For this review, take the finished solid that the model builds, in its own axes (mm). Face numbers are marked on the shaded views. A direction names the side the tool comes from. Round coordinates to 2 decimals unless told otherwise and drop trailing zeros. Order: outer loops, then holes, each group sorted by start corner. A loop starts at its lowest first (then second) coordinate and runs counter-clockwise, first axis right, second up. Notation, with made-up numbers: M 82,66.5 L 140,66.5 A29 cw 140,99.5 Z; hole C 3,-23.5 d2. An arc over 180 degrees is marked long. Use a Markdown table: item, result.
from build123d import *

# Parameters (mm, degrees)
F0_R          = 25.4
F0_R_2        = 12.7
F1_DEPTH      = 76.2
F3_START      = -12.7
F3_DEPTH      = 12.7
F4_DEPTH      = 12.7
F4_DEPTH_BACK = 25.4
F5_DEPTH      = 12.7
F5_DEPTH_BACK = 25.4
F6_DEPTH      = 76.201


with BuildPart() as f1:
    # F0 (on Right) → F1 (new body)
    with BuildSketch(Plane.YZ):
        Circle(F0_R)
        Circle(F0_R_2, mode=Mode.SUBTRACT)
    extrude(amount=F1_DEPTH)



with BuildPart() as f3:
    # F2 (on Front) → F3 (new body)
    with BuildSketch(Plane.XZ.offset(F3_START)):
        Polygon((0, 50.8), (0, 38.1), (10.16, 38.1), align=None)
    extrude(amount=-F3_DEPTH)


with BuildPart() as f1_1:
    add(f1.part)

    add(f3.part)  # F4 merges F3
    # F2 (on Front) → F4 (join, two sides)
    with BuildSketch(Plane.XZ) as f4_sk:
        Polygon((0, 38.1), (0, 22.5723106414), (21.9132695347, 22.5723106414), (10.16, 38.1), align=None)
    extrude(amount=F4_DEPTH)
    extrude(f4_sk.sketch, amount=-F4_DEPTH_BACK)

    # F2 (on Front) → F5 (join, two sides)
    with BuildSketch(Plane.XZ) as f5_sk:
        Polygon((0, 22.5723106414), (0, 0), (38.1, 0), (21.9132695347, 22.5723106414), align=None)
    extrude(amount=F5_DEPTH)
    extrude(f5_sk.sketch, amount=-F5_DEPTH_BACK)

    # F0 (on Right) → F6 (cut, through all)
    with BuildSketch(Plane.YZ):
        Circle(F0_R_2)
    extrude(amount=F6_DEPTH, mode=Mode.SUBTRACT)


solid = f1_1.part
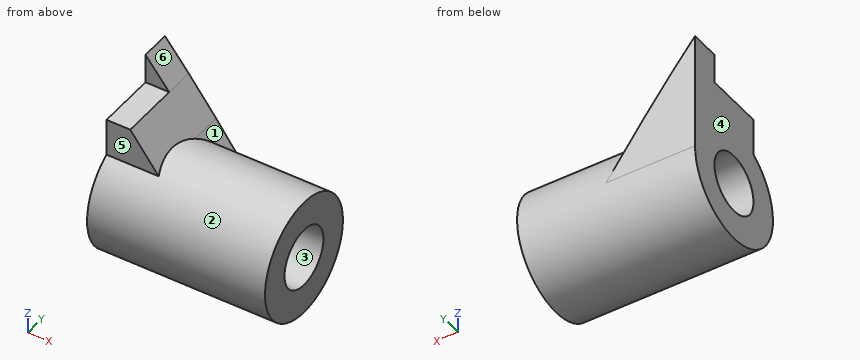
Q1. Add section A-A (y = 0). Write out the cut boundary in (x, z).
Determined:
| item | result |
|---|---|
| outline | M 0,-25.4 L 76.2,-25.4 L 76.2,-12.7 L 0,-12.7 Z; M 0,12.7 L 76.2,12.7 L 76.2,25.4 L 19.77,25.4 L 10.16,38.1 L 0,38.1 Z |
Q2. Clearance check with flat-ended pins moving along their axes: pin 1 (8 mm diameter, centred on x = 6, z = 45, fed in from -Y); pin 2 (1.5 mm diameter, centred on x = 14, z = 13.5, fed in from -Y); pin 3 (1 mm diameter, centred on x = 27.5, z = -14, fed in from -Y). State where each tip first meets the part, or that it passes through.
Determined:
| item | result |
|---|---|
| pin 1 | stops at y = 12.7 |
| pin 2 | stops at y = -21.97 |
| pin 3 | stops at y = -21.52 |
Q3. Add section D-D (z = 33). Write out the cut boundary in (x, y).
Determined:
| item | result |
|---|---|
| outline | M 0,-12.7 L 14.02,-12.7 L 14.02,25.4 L 0,25.4 Z |
Q4. Machinability: for the marked faces 5 and 6, which of the approach directions +Z, -Z, +X, -X, +Y, -Y give a long, thin tool a straight path to every point of the face, cutting with its end or side? Answer none if there is none.
Determined:
| item | result |
|---|---|
| face 5 | +Z, +X, -X, -Y |
| face 6 | +Z, +X, +Y, -Y |
Q5. Draft analysis for pull direction Z (two halves, no side actions). For the marked faces 1, 2, 3 and 4, state which applies: pulls with the +Z half, pulls with the -Z half, needs draft (parallel to the pull), parting line crosses it, or undercut.
Determined:
| item | result |
|---|---|
| face 1 | pulls with the +Z half |
| face 2 | parting line crosses it |
| face 3 | undercut |
| face 4 | needs draft |
Q6. Add section B-B (x = 62.5). Write out the cut boundary in (y, z), then the cut area to 3 significant figures.
Determined:
| item | result |
|---|---|
| outline | C 0,0 d50.8; hole C 0,0 d25.4 |
| area | 1,520 mm^2 |
Q7. Wall thickness on line 1 along Z through (x, y) = (31, 0); line 2 along Y through (x, z) = (46, -0.5); line 3 along Y through (x, z) = (9.5, 36.5): over which ranges is each line inside the solid? List them lowest first. Write a range as [from, to].
Determined:
| item | result |
|---|---|
| line 1 | z = [-25.4, -12.7], [12.7, 25.4] |
| line 2 | y = [-25.4, -12.69], [12.69, 25.4] |
| line 3 | y = [-12.7, 25.4] |
Q8. Add section C-C (y = -19.5). Write out the cut boundary in (x, z), then the cut area to 3 significant figures.
Determined:
| item | result |
|---|---|
| outline | M 0,-16.28 L 76.2,-16.28 L 76.2,16.28 L 0,16.28 Z |
| area | 2,480 mm^2 |
